Check sheet for the modelled part. Datum: model origin and axes. Units: mm. A direction names the side the tool comes from. Round coordinates to 2 decimals unless told otherwise and drop trailing zeros. Loops run counter-clockwise (first coordinate to the right, second up) from the corner with the lowest first, then second, coordinate; pieces in that order, holes last. Notation, with made-up numbers: M 50,11 L 84,11 A32 cw 84,47 Z; hole C 64,27.5 d10. An arc over 180 degrees is marked long. Write item = value, one per line. Start each with the question number.
(1) Cross-section at C-C on z = -9.75. Record the boundary of the cut face in (x, y).
(2) Go/stop test with flat-tipped pins: P1, Ø3, axis at x = 6, z = 2, coming from the +Y side; P2, Ø1, axis at y = 7, z = 2.5, coming from the +X side; P3, Ø5, axis at y = 5, z = -8.5, coming from the -X side. Record where each tip stops, or that it passes through.
(3) Set-up check for faces 1 (the face through (0, 5.5, 3)), 2 (the face through (-10.1, 0, 0)), 3 (the face through (-3.3, 3, 3)): record each of +Z, -Z, +X, -X, +Y, -Y from which the full face is reachable in a straight line by a thin tool's end or side.
(4) Scan lines: L1, parallel to Y at x = 21, z = 0; L2, parallel to X at y = 7.75, z = 8.75; L3, parallel to Y at x = -3, z = 6.25. Record each from-to range of solid material in increasing order. Write a range as from..to.
(5) Cross-section at D-D on x = 21.5. Record the boundary of the cut face in (y, z), plus the area to 3 significant figures.
(6) Cross-section at B-B on z = 0. Record the boundary of the cut face in (x, y) (3 decimals), plus the area to 3 significant figures.
from build123d import *

# Parameters (mm, degrees)
SKETCH1_W          = 6.8
SKETCH1_H          = 3.133597909
SKETCH1_W_2        = 20.655905863
SKETCH1_W_3        = 7.244094137
SKETCH2_R          = 1.59
CUT_EXTRUDE1_DEPTH = 10
CIRPATTERN1_COUNT  = 3
CHAMFER1_SIZE      = 0.4


with BuildPart() as part:
    # Sketch1 → Revolve1 (revolve)
    with BuildSketch(Plane.XY, mode=Mode.PRIVATE) as revolve1_sk:
        with Locations((-6.7, 1.566798955)):
            Rectangle(SKETCH1_W, SKETCH1_H)
        with Locations((7.027952931, 1.566798955)):
            Rectangle(SKETCH1_W_2, SKETCH1_H)
        Polygon((17.355905863, 3.133597909), (17.355905863, 6.095), (12.7, 6.095), (12.7, 5.859469346), (12.242129105, 5.859469346), (12.242129105, 6.107765985), (0, 6.107765985), (0, 12.7), (-3.3, 12.7), (-3.3, 3.133597909), align=None)
        with Locations((20.977952931, 1.566798955)):
            Rectangle(SKETCH1_W_3, SKETCH1_H)
    revolve(revolve1_sk.sketch.rotate(Axis((-3.3, 0, 0), (1, 0, 0)), 90), axis=Axis((-3.3, 0, 0), (1, 0, 0)))

    # Sketch2 → Cut-Extrude1 (cut)
    with BuildSketch(Plane(origin=(0, 0, 0), x_dir=(0, 0, -1), z_dir=(1, 0, 0))):
        with Locations((9.75, 0)):
            Circle(SKETCH2_R)
    cut_extrude1 = extrude(amount=-CUT_EXTRUDE1_DEPTH, mode=Mode.SUBTRACT)

    # CirPattern1: Cut-Extrude1 ×3 about axis
    cirpattern1_axis = Axis((0, 0, 0), (1, 0, 0))
    for i in range(1, CIRPATTERN1_COUNT):
        add(cut_extrude1.rotate(cirpattern1_axis, i * 360 / CIRPATTERN1_COUNT), mode=Mode.SUBTRACT)

    # Chamfer1
    # the kernel refuses this chamfer: 0.4 mm, written as the material it takes off along each edge
    with BuildSketch(Plane(origin=(17.355905863, 0, 0), x_dir=(0, 0, 1), z_dir=(0, 1, 0))) as chamfer1_piece_1:
        Polygon((6.095, -CHAMFER1_SIZE), (6.095 - CHAMFER1_SIZE, 0), (6.095, 0), align=None)
    revolve(axis=Axis((17.355905863, 0, 0), (1, 0, 0)), mode=Mode.SUBTRACT)
    with BuildSketch(Plane(origin=(12.7, 0, 0), x_dir=(0, 0, 1), z_dir=(0, 1, 0))) as chamfer1_piece_2_section:
        Polygon((6.095 - CHAMFER1_SIZE, 0), (6.095, CHAMFER1_SIZE), (6.095, 0), align=None)
    chamfer1_piece_2 = revolve(axis=Axis((12.7, 0, 0), (1, 0, 0)), mode=Mode.PRIVATE)
    chamfer1_piece_2 = chamfer1_piece_2 - Plane(origin=(12.978018591, 0, 0), x_dir=(0, 0, 1), z_dir=(-1, 0, 0)) * Cylinder(5.859469346, 25, mode=Mode.PRIVATE)
    add(chamfer1_piece_2, mode=Mode.SUBTRACT)
    with BuildSketch(Plane(origin=(12.242129105, 0, 0), x_dir=(0, 0, 1), z_dir=(0, 1, 0))) as chamfer1_piece_3_section:
        Polygon((6.107765985, -CHAMFER1_SIZE), (6.107765985 - CHAMFER1_SIZE, 0), (6.107765985, 0), align=None)
    chamfer1_piece_3 = revolve(axis=Axis((12.242129105, 0, 0), (1, 0, 0)), mode=Mode.PRIVATE)
    chamfer1_piece_3 = chamfer1_piece_3 - Plane(origin=(11.970594619, 0, 0), x_dir=(0, 0, 1), z_dir=(-1, 0, 0)) * Cylinder(5.859469346, 25, mode=Mode.PRIVATE)
    add(chamfer1_piece_3, mode=Mode.SUBTRACT)


solid = part.part
Result:
q1.outline = M -3.3,-8.14 L 0,-8.14 L 0,-1.59 L -3.3,-1.59 Z; M -3.3,1.59 L 0,1.59 L 0,8.14 L -3.3,8.14 Z
q2.P1 = 6.09
q2.P2 = 0
q2.P3 = -3.3
q3.face_1 = +X
q3.face_2 = +Z, -Z, -X, +Y, -Y
q3.face_3 = -X
q4.L1 = -3.13..3.13
q4.L2 = -3.3..0
q4.L3 = -11.06..-9.24, -7.65..7.65, 9.24..11.06
q5.outline = C 0,0 d6.27
q5.area = 30.8 mm^2
q6.outline = M -10.1,-3.134 L -3.3,-3.134 L -3.3,-12.7 L 0,-12.7 L 0,-6.108 L 11.842,-6.108 L 12.09,-5.859 L 12.864,-5.859 L 13.1,-6.095 L 16.956,-6.095 L 17.356,-5.695 L 17.356,-3.134 L 24.6,-3.134 L 24.6,3.134 L 17.356,3.134 L 17.356,5.695 L 16.956,6.095 L 13.1,6.095 L 12.864,5.859 L 12.09,5.859 L 11.842,6.108 L 0,6.108 L 0,12.7 L -3.3,12.7 L -3.3,3.134 L -10.1,3.134 Z
q6.area = 383 mm^2
